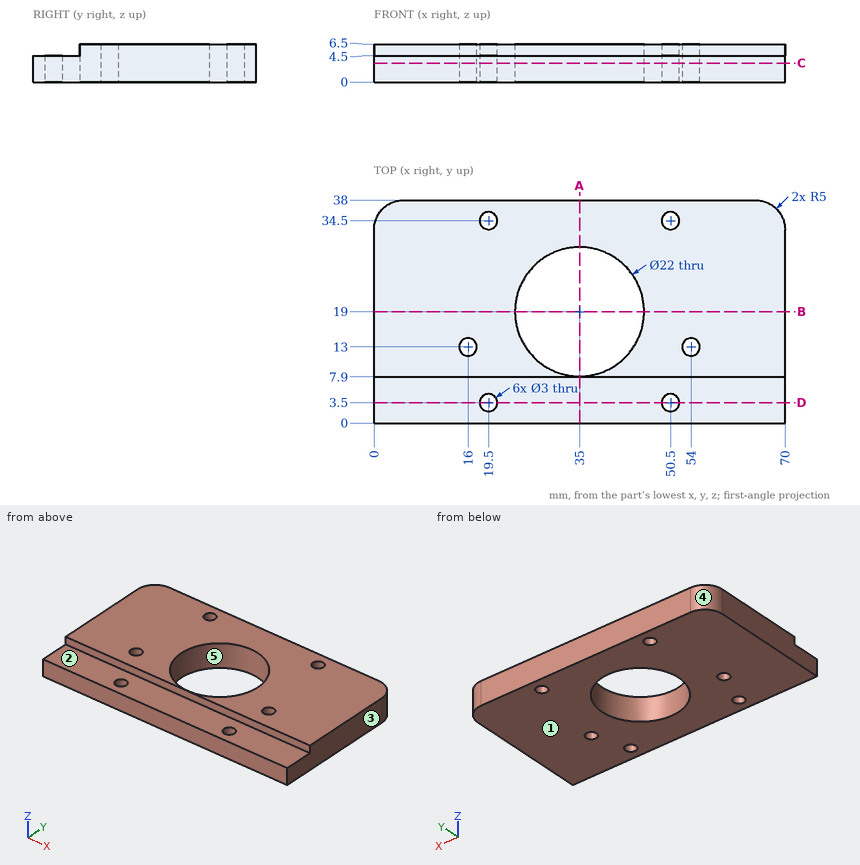
Drawing for the job (mm, zero at the part's lowest x, y, z). A direction names the side the tool comes from. Round coordinates to 2 decimals unless told otherwise and drop trailing zeros. Write each loop counter-clockwise with the first axis right and the second up, starting at its lowest first coordinate (ties: lowest second). Pieces come first, ordered by that corner, then holes. Notation, with made-up numbers: (-6.75, 34) - (18.25, 34) arc R18 ccw to (18.25, 63) - close; hole circle Ø1 at (-27, -9). An arc over 180 degrees is marked (long way). Write item = value, one per line. Start each with the question number.
Q1. Band-saw the part on C-C (z = 3.25). Give the cut face in (x, y).
Q2. Band-saw the part on D-D (y = 3.5). Give the cut face in (x, z), then the cut area to 3 significant figures.
Q3. Drop flat-ended pins along their axis: pin 1 (6.5 mm diameter, centred on x = 52, y = 2.5, fed in from +Z); pin 2 (2.5 mm diameter, centred on x = 19.5, y = 3.5, fed in from +Z); pin 3 (2 mm diameter, centred on x = 47, z = 6, fed in from -Y). Give the stop position or say it passes through.
Q4. Band-saw the part on A-A (x = 35). Give the cut face in (y, z).
Q5. Which spindle directions (+Z, -Z, +X, -X, +Y, -Y) get a long thin tool onto all of the face, cutting with end or side? Do the marked faces 1 and 2. Say none if no direction does.
Q6. Mould opens along Y. For the marked faces 3, 4 and 5 say: pulls with the +Y half, pulls with the -Y half, needs draft (parallel to the pull), parting line crosses it, or undercut.
Q7. Probe L1, parallel to Y at x = 50.5, z = 3.3; L2, parallel to X at y = 18.5, z = 3.75; L3, parallel to X at y = 2.5, z = 3.5. List the from-to ranges inside material, lowest first. Write a range as from..to.
Q8. Band-saw the part on B-B (y = 19). Give the cut face in (x, z).
Answers below:
q1.outline = (0, 0) - (70, 0) - (70, 33) arc R5 ccw to (65, 38) - (5, 38) arc R5 ccw to (0, 33) - close; hole circle Ø3 at (16, 13); hole circle Ø3 at (19.5, 3.5); hole circle Ø3 at (19.5, 34.5); hole circle Ø22 at (35, 19); hole circle Ø3 at (50.5, 3.5); hole circle Ø3 at (50.5, 34.5); hole circle Ø3 at (54, 13)
q2.outline = (0, 0) - (18, 0) - (18, 4.5) - (0, 4.5) - close; (21, 0) - (49, 0) - (49, 4.5) - (21, 4.5) - close; (52, 0) - (70, 0) - (70, 4.5) - (52, 4.5) - close
q2.area = 288 mm2
q3.pin_1 = 4.5
q3.pin_2 = through
q3.pin_3 = 7.9
q4.outline = (0, 0) - (8, 0) - (8, 6.5) - (7.9, 6.5) - (7.9, 4.5) - (0, 4.5) - close; (30, 0) - (38, 0) - (38, 6.5) - (30, 6.5) - close
q5.face_1 = -Z, +X, -X, +Y, -Y
q5.face_2 = +Z, +X, -X, -Y
q6.face_3 = needs draft
q6.face_4 = pulls with the +Y half
q6.face_5 = undercut
q7.L1 = 0..2, 5..33, 36..38
q7.L2 = 0..24.01, 45.99..70
q7.L3 = 0..18.38, 20.62..49.38, 51.62..70
q8.outline = (0, 0) - (24, 0) - (24, 6.5) - (0, 6.5) - close; (46, 0) - (70, 0) - (70, 6.5) - (46, 6.5) - close
